Can you work these out from the model? Positions are in its coordinate system, mm. A direction names the side the tool comes from. Give positions to 0.01 mm unless a question says otherwise; leave off trailing zeros. Loops run counter-clockwise (first coordinate to the right, second up) from the corner with the lowest first, then second, coordinate; pieces in that order, holes last. Notation, with made-up numbers: (4, -1.75) -> (25, -1.75) arc R28 cw to (25, 23.25) -> close; hole circle Ø10 at (62.5, -39). An arc over 180 degrees is marked (long way). Return JSON: item names as keys, results as strings. Group by question number.
Q1. Which directions (+Z, -Z, +X, -X, +Y, -Y) give clear straight access to the entire face, cutting with the end or side of a thin tool? Please do faces 5 (the flat face through (52, 7, -30.6)), 6 (the flat face through (83.588, 0.986, -30.066)).
Q2. Suppose I cut it at B-B, the plane y = 8.5. Please give me the cut outline in (x, z), and give its area (3 significant figures).
Q3. Suppose I cut it at D-D, the plane x = 82.75. Please give me the cut outline in (y, z), and give its area (3 significant figures).
Q4. I need wall thicknesses on line 1 along X through (y, z) = (1.3, -6.6); line 2 along Z through (x, y) = (30, 9); line 3 along Y through (x, z) = (26, -27.5). Which ranges of each line are inside material? Lowest first, please. Write a range as [from, to].
Q5. Will these pins go through, and if not, where does the flat tip stop? pin 1 (6.5 mm diameter, centred on x = 64.75, y = 8.5, fed in from +Z); pin 2 (9 mm diameter, centred on x = 13, z = -18.6, fed in from +Y); pin 3 (0.6 mm diameter, centred on x = 67.5, y = 1.5, fed in from +Z).
Q6. Suppose I cut it at A-A, the plane x = 61. Please give me the cut outline in (y, z).
Q7. Thinking about a two-plate mould opening in Z: for faces 1 (the cylindrical face through (77.8, 1.01, -17.43)), 2 (the flat face through (93.75, 1, -14)), 3 (the flat face through (77.737, 0.986, -7.148)), 4 (the cylindrical face through (84.237, 0.986, -6.795)), which applies, pulls with the +Z half, pulls with the -Z half, needs draft (parallel to the pull), parting line crosses it, or undercut?
Q8. Suppose I cut it at C-C, the plane z = -16. Please give me the cut outline in (x, y).
```python
from build123d import *

# Parameters (mm, degrees)
SKETCH1_R           = 1.5
SKETCH1_R_2         = 4
SKETCH1_W           = 31.5
SKETCH1_H           = 6.5
BOSS_EXTRUDE1_DEPTH = 2
SKETCH2_W           = 52.75
SKETCH2_H           = 2
BOSS_EXTRUDE2_DEPTH = 10
SKETCH3_R           = 2
CUT_EXTRUDE1_DEPTH  = 100.1617996
FILLET1_R           = 1.5
FILLET2_R           = 1
FILLET3_R           = 1.5


with BuildPart() as part:
    # Sketch1 → Boss-Extrude1 (new body)
    with BuildSketch(Plane(origin=(0, 0, 0), x_dir=(1, 0, 0), z_dir=(0, 1, 0))):
        Polygon((0, 5.6), (30, 5.6), (33, 2.6), (44, 2.6), (47, 11.6), (76.5, 11.6), (79, 2.6), (90, 2.6), (93.75, 8.1), (93.75, 19.6), (88.25, 29.6), (78.25, 30.6), (78.25, 32.6), (25.5, 32.6), (25.5, 30.6), (0, 24.6), align=None)
        with Locations(Location((82.75, 6.6, 0), (0, 0, 270))):
            Circle(SKETCH1_R, mode=Mode.SUBTRACT)
        with Locations(Location((38, 6.6, 0), (0, 0, 270))):
            Circle(SKETCH1_R, mode=Mode.SUBTRACT)
        with Locations(Location((13, 18.6, 0), (0, 0, 270))):
            Circle(SKETCH1_R_2, mode=Mode.SUBTRACT)
        with Locations(Location((29, 18.6, 0), (0, 0, 270))):
            Circle(SKETCH1_R_2, mode=Mode.SUBTRACT)
        with Locations((62.5, 20.25)):
            Rectangle(SKETCH1_W, SKETCH1_H, mode=Mode.SUBTRACT)
    extrude(amount=BOSS_EXTRUDE1_DEPTH)

    # Sketch2 → Boss-Extrude2 (add)
    with BuildSketch(Plane(origin=(0, 2, 0), x_dir=(1, 0, 0), z_dir=(0, 1, 0))):
        with Locations((51.875, 31.6)):
            Rectangle(SKETCH2_W, SKETCH2_H)
    extrude(amount=BOSS_EXTRUDE2_DEPTH)

    # Sketch3 → Cut-Extrude1 (cut, through all)
    with BuildSketch(Plane(origin=(0, 0, -32.6), x_dir=(-1, 0, 0), z_dir=(0, 0, -1))):
        with Locations((-64.75, 8.5)):
            Circle(SKETCH3_R)
        with Locations((-39.75, 8.5)):
            Circle(SKETCH3_R)
    extrude(amount=-CUT_EXTRUDE1_DEPTH, mode=Mode.SUBTRACT)

    # Fillet1
    fillet1_edges = [part.edges().sort_by_distance(p)[0] for p in [
        (46.75, 1, -17),
        (46.75, 1, -23.5),
        (0, 1, -24.6),
        (25.5, 1, -30.6),
        (25.5, 12, -31.6),
        (78.25, 1, -17),
        (78.25, 1, -23.5),
        (0, 1, -5.6),
        (30, 1, -5.6),
        (33, 1, -2.6),
        (44, 1, -2.6),
        (47, 1, -11.6),
        (76.5, 1, -11.6),
        (79, 1, -2.6),
        (90, 1, -2.6),
        (93.75, 1, -8.1),
        (93.75, 1, -19.6),
        (88.25, 1, -29.6),
        (78.25, 1, -30.6),
        (78.25, 12, -31.6),
    ]]
    fillet(fillet1_edges, radius=FILLET1_R)

    # Fillet2
    fillet2_edges = [part.edges().sort_by_distance(p)[0] for p in [
        (51.875, 2, -30.6),
    ]]
    fillet(fillet2_edges, radius=FILLET2_R)

    # Fillet3
    fillet3_edges = [part.edges().sort_by_distance(p)[0] for p in [
        (51.875, 0, -32.6),
    ]]
    fillet(fillet3_edges, radius=FILLET3_R)


solid = part.part
```
Ans:
{
 "1": {"face 5": "+Z, +X, -X, +Y", "face 6": "-Z, +X, +Y, -Y"},
 "2": {"outline": "(25.5, -32.6) -> (37.75, -32.6) -> (37.75, -30.6) -> (25.5, -30.6) -> close; (41.75, -32.6) -> (62.75, -32.6) -> (62.75, -30.6) -> (41.75, -30.6) -> close; (66.75, -32.6) -> (78.25, -32.6) -> (78.25, -30.6) -> (66.75, -30.6) -> close", "area": "89.5 mm^2"},
 "3": {"outline": "(0, -30.15) -> (2, -30.15) -> (2, -8.1) -> (0, -8.1) -> close; (0, -5.1) -> (2, -5.1) -> (2, -2.6) -> (0, -2.6) -> close", "area": "49.1 mm^2"},
 "4": {"line 1": "x = [0.09, 36.5], [39.5, 45.33], [77.89, 81.25], [84.25, 92.73]", "line 2": "z = [-32.6, -30.6]", "line 3": "y = [0, 2]"},
 "5": {"pin 1": "stops at z = -30.6", "pin 2": "stops at y = 2", "pin 3": "stops at z = -11.6"},
 "6": {"outline": "(0, -31.1) arc R1.5 ccw to (1.5, -32.6) -> (12, -32.6) -> (12, -30.6) -> (3, -30.6) arc R1 cw to (2, -29.6) -> (2, -23.5) -> (0, -23.5) -> close; (0, -17) -> (2, -17) -> (2, -11.6) -> (0, -11.6) -> close"},
 "7": {"face 1": "undercut", "face 2": "needs draft", "face 3": "pulls with the +Z half", "face 4": "undercut"},
 "8": {"outline": "(0, 0) -> (9.96, 0) -> (9.96, 2) -> (0, 2) -> close; (16.04, 0) -> (25.96, 0) -> (25.96, 2) -> (16.04, 2) -> close; (32.04, 0) -> (93.75, 0) -> (93.75, 2) -> (32.04, 2) -> close"}
}
